Can you work these out from the model? Positions are in its coordinate system, mm. Give positions to 0.01 mm unless a question says otherwise; leave off trailing zeros. Order: outer loops, then holes, each group sorted by start corner. A loop starts at its lowest first (then second) coordinate and runs counter-clockwise, first axis right, second up. Notation, with made-up numbers: (50, 62) - (81, 62) arc R23 ccw to (81, 101) - close; hole circle Ø4 at (74, 63.5). An arc over 180 degrees is marked (long way). Answer as CSV lines item,"result".
```python
from build123d import *

# Parameters (mm, degrees)
SKETCH_1_W          = 5.1
SKETCH_1_H          = 0.8
CUT_EXTRUDE_1_DEPTH = 8.256721023
FILLET_1_R          = 0.15


with BuildPart() as part:
    # 草图1 → 旋转1 (revolve)
    with BuildSketch(Plane.XY):
        with Locations((2.55, 68.708527966)):
            Rectangle(SKETCH_1_W, SKETCH_1_H)
    revolve(axis=Axis((0, 69.108527966, 0), (0, -1, 0)))

    # 草图2 → 切除-拉伸1 (cut, through all)
    with BuildSketch(Plane(origin=(0, 69.108527966, 0), x_dir=(-1, 0, 0), z_dir=(0, 1, 0))):
        with BuildLine():
            Line((-3.199553455, 0.570374573), (-3.918273635, 0.804424081))
            ThreePointArc((-3.918273635, 0.804424081), (-3.994373733, 0.21199127), (-3.981407211, -0.385168448))
            Line((-3.981407211, -0.385168448), (-3.241952523, -0.228501177))
            ThreePointArc((-3.241952523, -0.228501177), (-3.139811906, -0.839077143), (-2.923750279, -1.419209101))
            Line((-2.923750279, -1.419209101), (-3.642772796, -1.65232263))
            ThreePointArc((-3.642772796, -1.65232263), (-3.356118206, -2.176334942), (-2.994630559, -2.651820418))
            Line((-2.994630559, -2.651820418), (-2.488484708, -2.090434413))
            ThreePointArc((-2.488484708, -2.090434413), (-2.046963571, -2.524364167), (-1.531172889, -2.866703062))
            Line((-1.531172889, -2.866703062), (-1.975859509, -3.477924527))
            ThreePointArc((-1.975859509, -3.477924527), (-1.435936071, -3.733365668), (-0.863994936, -3.905559842))
            Line((-0.863994936, -3.905559842), (-0.784496864, -3.153893672))
            ThreePointArc((-0.784496864, -3.153893672), (-0.172242423, -3.245430066), (0.446261515, -3.219213824))
            Line((0.446261515, -3.219213824), (0.445759758, -3.975082601))
            ThreePointArc((0.445759758, -3.975082601), (1.032712913, -3.864387477), (1.596638706, -3.667524283))
            Line((1.596638706, -3.667524283), (1.219138949, -3.012671786))
            ThreePointArc((1.219138949, -3.012671786), (1.768268328, -2.726851874), (2.253240152, -2.342094254))
            Line((2.253240152, -2.342094254), (2.697131397, -2.953893593))
            ThreePointArc((2.697131397, -2.953893593), (3.106915443, -2.519331172), (3.447420884, -2.028593455))
            Line((3.447420884, -2.028593455), (2.75711029, -1.720709844))
            ThreePointArc((2.75711029, -1.720709844), (3.033363561, -1.166707614), (3.199558641, -0.570374203))
            Line((3.199558641, -0.570374203), (3.918278822, -0.80442371))
            ThreePointArc((3.918278822, -0.80442371), (3.994378087, -0.211986219), (3.981409517, 0.385177991))
            Line((3.981409517, 0.385177991), (3.241957709, 0.228501547))
            ThreePointArc((3.241957709, 0.228501547), (3.139817092, 0.83907751), (2.923755466, 1.419209465))
            Line((2.923755466, 1.419209465), (3.642783633, 1.65231108))
            ThreePointArc((3.642783633, 1.65231108), (3.356126982, 2.176329766), (2.994635746, 2.651820782))
            Line((2.994635746, 2.651820782), (2.488489895, 2.090434778))
            ThreePointArc((2.488489895, 2.090434778), (2.046968759, 2.524364531), (1.531178079, 2.866703425))
            Line((1.531178079, 2.866703425), (1.975864699, 3.477924889))
            ThreePointArc((1.975864699, 3.477924889), (1.435941262, 3.733366031), (0.864000127, 3.905560207))
            Line((0.864000127, 3.905560207), (0.784502055, 3.153894037))
            ThreePointArc((0.784502055, 3.153894037), (0.172247613, 3.245430432), (-0.446256324, 3.21921419))
            Line((-0.446256324, 3.21921419), (-0.445754567, 3.975082967))
            ThreePointArc((-0.445754567, 3.975082967), (-1.032707749, 3.864387836), (-1.596633567, 3.667524629))
            Line((-1.596633567, 3.667524629), (-1.219133759, 3.012672153))
            ThreePointArc((-1.219133759, 3.012672153), (-1.768263138, 2.726852242), (-2.253234963, 2.342094623))
            Line((-2.253234963, 2.342094623), (-2.697126207, 2.953893962))
            ThreePointArc((-2.697126207, 2.953893962), (-3.106910254, 2.519331541), (-3.447415696, 2.028593825))
            Line((-3.447415696, 2.028593825), (-2.757105101, 1.720710213))
            ThreePointArc((-2.757105101, 1.720710213), (-3.033358374, 1.166707983), (-3.199553455, 0.570374573))
        make_face()
    extrude(amount=-CUT_EXTRUDE_1_DEPTH, mode=Mode.SUBTRACT)

    # 圆角1
    fillet_1_edges = [part.edges().sort_by_distance(p)[0] for p in [
        (-5.1, 68.308527966, 0),
        (-5.1, 69.108527966, 0),
    ]]
    fillet(fillet_1_edges, radius=FILLET_1_R)


solid = part.part
```
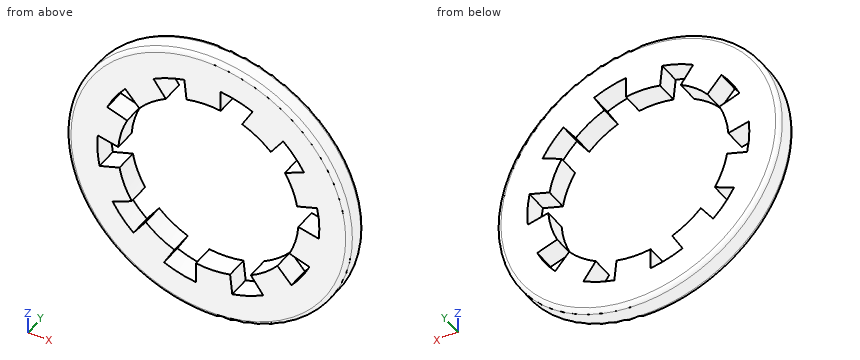
1) I want a section at A-A on x = 0. Write out the boundary of the cut face in (y, z).
Answer block:
outline,"(68.31, -4.95) arc R0.15 ccw to (68.46, -5.1) - (68.96, -5.1) arc R0.15 ccw to (69.11, -4.95) - (69.11, -3.25) - (68.31, -3.25) - close; (68.31, 3.25) - (69.11, 3.25) - (69.11, 4.95) arc R0.15 ccw to (68.96, 5.1) - (68.46, 5.1) arc R0.15 ccw to (68.31, 4.95) - close"
2) I need wall thicknesses on line 1 along X through (y, z) = (69.05, 2.5); line 2 along Z through (x, y) = (-0.25, 68.9); line 3 along Z through (x, y) = (1.5, 68.6). Which ranges of each line are inside material? Lowest first, please. Write a range as [from, to].
Answer block:
line 1,"[-4.41, -3.12], [-2.86, -2.08], [2.08, 2.37], [3.12, 4.41]"
line 2,"[-5.09, -3.24], [3.24, 5.09]"
line 3,"[-4.87, -3.71], [2.88, 3.5], [3.71, 4.87]"
3) I want a section at B-B on z = 0. Write out the boundary of the cut face in (x, y), plus the area to 3 significant figures.
Answer block:
outline,"(-5.1, 68.46) arc R0.15 ccw to (-4.95, 68.31) - (-4, 68.31) - (-4, 69.11) - (-4.95, 69.11) arc R0.15 ccw to (-5.1, 68.96) - close; (4, 68.31) - (4.95, 68.31) arc R0.15 ccw to (5.1, 68.46) - (5.1, 68.96) arc R0.15 ccw to (4.95, 69.11) - (4, 69.11) - close"
area,"1.74 mm2"
